Source: CAD feature listing. Evaluate the final solid. Frame: model axes, mm. Give positions to 0.01 mm unless a question says otherwise; leave off trailing zeros. Order: outer loops, then holes, each group sorted by start corner. A loop starts at its lowest first (then second) coordinate and runs counter-clockwise, first axis right, second up. Notation, with made-up numbers: M 43,46.25 L 74,46.25 A11 cw 74,67.25 Z; hole C -3,-26 d1. An arc over 180 degrees is marked long. One line per question, with ' | ' between items. Start each with the question number.
from build123d import *

# Parameters (mm, degrees)
SKETCH1_W            = 400
SKETCH1_H            = 280
BOSS_EXTRUDE1_DEPTH  = 6.35
CHAMFER1_SIZE        = 25
SKETCH2_R            = 12.5
CUT_EXTRUDE1_DEPTH   = 489.303514732
M6_CLEARANCE_HOLE1_D = 6.6


with BuildPart() as part:
    # Sketch1 → Boss-Extrude1 (new body)
    with BuildSketch(Plane(origin=(0, 0, 0), x_dir=(1, 0, 0), z_dir=(0, 1, 0))):
        with Locations((200, 140)):
            Rectangle(SKETCH1_W, SKETCH1_H)
    extrude(amount=BOSS_EXTRUDE1_DEPTH)

    # Chamfer1
    chamfer1_edges = [part.edges().sort_by_distance(p)[0] for p in [
        (0, 3.175, -280),
        (400, 3.175, -280),
        (400, 3.175, 0),
        (0, 3.175, 0),
    ]]
    chamfer(chamfer1_edges, length=CHAMFER1_SIZE)

    # Sketch2 → Cut-Extrude1 (cut, through all)
    with BuildSketch(Plane(origin=(0, 6.35, 0), x_dir=(1, 0, 0), z_dir=(0, 1, 0))):
        with Locations(Location((349.2, 140, 0), (0, 0, 270))):
            Circle(SKETCH2_R)
    extrude(amount=-CUT_EXTRUDE1_DEPTH, mode=Mode.SUBTRACT)

    # M6 Clearance Hole1 (through all)
    with Locations(Plane(origin=(0, 6.35, 0), x_dir=(1, 0, 0), z_dir=(0, 1, 0))):
        with Locations((380, 230), (380, 50), (20, 50), (20, 230)):
            Hole(M6_CLEARANCE_HOLE1_D / 2)


solid = part.part
Item 1: Cut plane C-C on z = -135. Return the cut outline in (x, y).
Item 2: Cut plane B-B on x = 349.2. Return the cut outline in (y, z), and give its area (3 significant figures).
Item 3: Mould query, pull axis Z, two halves, no side actions, for faces 1 (the flat face through (13, 3, -12)), 2 (the flat face through (197, 0, -142)), 3 (the cylindrical face through (359.74, 3.22, -133.28)), 4 (the flat face through (387, 3, -268)). Classes: pulls with the +Z half, pulls with the -Z half, needs draft (parallel to the pull), parting line crosses it, or undercut.
Item 4: Cut plane A-A on y = 4.5. Return the cut outline in (x, z), and give its area (3 significant figures).
Item 5: Line query: line 1 (X direction, y = 3.5, z = -50); line 2 (X direction, y = 3.25, z = -139.5); line 3 (Z direction, x = 20, y = 3.25). Output: solid intervals per line, ascending.
Results are:
1) outline: M 0,0 L 337.74,0 L 337.74,6.35 L 0,6.35 Z; M 360.66,0 L 400,0 L 400,6.35 L 360.66,6.35 Z
2) outline: M 0,-280 L 6.35,-280 L 6.35,-152.5 L 0,-152.5 Z; M 0,-127.5 L 6.35,-127.5 L 6.35,0 L 0,0 Z | area: 1,620 mm2
3) face 1: pulls with the +Z half | face 2: needs draft | face 3: undercut | face 4: pulls with the -Z half
4) outline: M 0,-255 L 25,-280 L 375,-280 L 400,-255 L 400,-25 L 375,0 L 25,0 L 0,-25 Z; hole C 20,-230 d6.6; hole C 20,-50 d6.6; hole C 349.2,-140 d25; hole C 380,-230 d6.6; hole C 380,-50 d6.6 | area: 110,000 mm2
5) line 1: x = 0 to 16.7, 23.3 to 376.7, 383.3 to 400 | line 2: x = 0 to 336.71, 361.69 to 400 | line 3: z = -275 to -233.3, -226.7 to -53.3, -46.7 to -5
